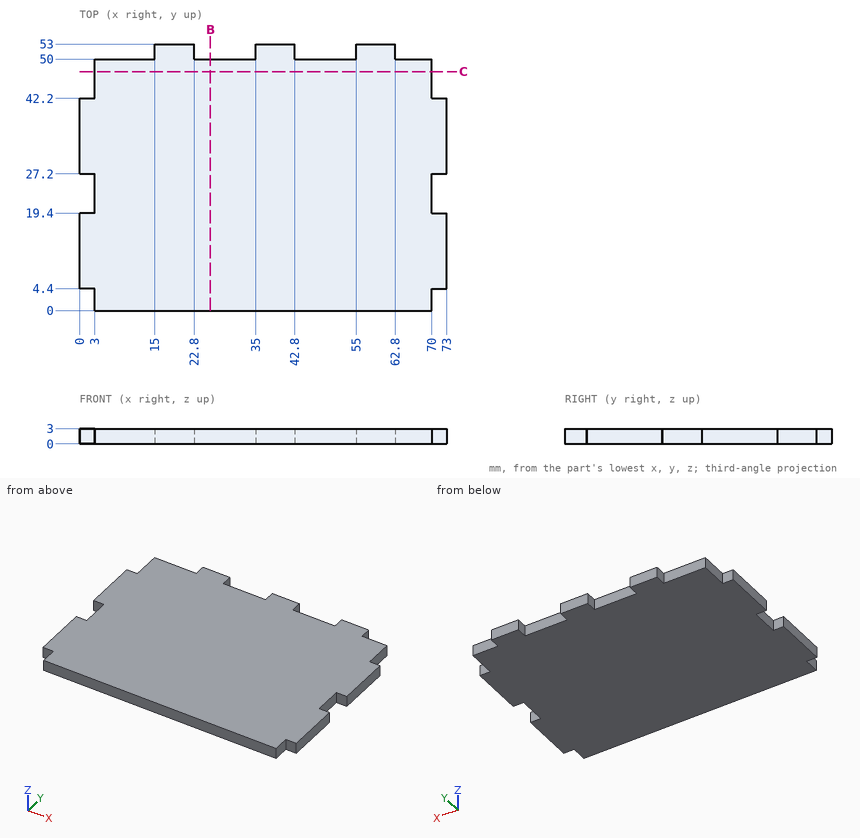
Design review of the part shown in the three views and the two pictorial views. Dimensions are in mm from the part's minimum x, y and z. Give positions to 0.01 mm unless a question says otherwise; leave off trailing zeros. Loops run counter-clockwise (first coordinate to the right, second up) from the corner with the lowest first, then second, coordinate; pieces in that order, holes last. Notation, with made-up numbers: M 88.25,69 L 118.25,69 A26 cw 118.25,90 Z; hole C 19,55.25 d7. An arc over 180 degrees is marked long. Answer as a JSON object with one key per item and string values. Group by question number.
Q1. Add section B-B on x = 26. Give the boundary of the cut face in (y, z).
Q2. Add section C-C on y = 47.5. Give the boundary of the cut face in (x, z), and give its area (3 significant figures).
Q3. Insertion check: P1, Ø1.5, axis at x = 72, z = 1, coming from the -Y side; P2, Ø1.5, axis at y = 51.5, z = 1, coming from the +X side; P3, Ø0.9, axis at x = 29, z = 2, coming from the +Y side. Each pin has a flat end and moves straight along its axis. Give the tip position at first contact, or say it passes through.
Q4. For probe 1 along Y at (x, z) = (70.5, 2.15); probe 2 along Y at (x, z) = (9, 2.15); probe 3 along X at (y, z) = (44, 0.4), list the stretches that pass through material, from the lowest coordinate up. Write a range as [from, to].
Checked values:
{
 "1": {"outline": "M 0,0 L 50,0 L 50,3 L 0,3 Z"},
 "2": {"outline": "M 3,0 L 70,0 L 70,3 L 3,3 Z", "area": "201 mm²"},
 "3": {"P1": "y = 4.4", "P2": "x = 62.8", "P3": "y = 50"},
 "4": {"probe 1": "[4.4, 19.4], [27.2, 42.2]", "probe 2": "[0, 50]", "probe 3": "[3, 70]"}
}
